```python
from build123d import *

# Parameters (mm, degrees)
F1_DEPTH      = 3
F2_DEPTH      = 6.85
F6_DEPTH      = 3
F3_W          = 16.2
F3_H          = 1
F7_DEPTH      = 1
F5_W          = 16.2
F5_H          = 1
F8_DEPTH      = 1
F4_W          = 1
F4_H          = 18.8
F9_DEPTH      = 1
F0_W          = 7
F0_H          = 10
F10_DEPTH     = 3
F11_D         = 8.2
F12_D         = 5
F13_R         = 0.6
F14_R         = 0.6
F15_T1_DEPTH  = 18
F15_S5_W      = 0.6
F15_S5_H      = 0.6
F15_T6_DEPTH  = 0.6
F15_S11_W     = 0.6
F15_S11_H     = 0.6
F15_T12_DEPTH = 0.6


# Not quite as in the source:
# - a fillet or chamfer that OpenCascade refuses, or shapes differently, is made with other operations: its cross-section is extruded or revolved along the edge and cut away or added
# - a feature names something its author has since deleted; it is built from what else it names


with BuildPart() as f1:
    # F0 (on Front) → F1 (new body)
    with BuildSketch(Plane.XZ):
        Polygon((0.9, 2.1), (4.9, 2.1), (21.1, 2.1), (21.1, 20.9), (4.9, 20.9), (0.9, 20.9), align=None)
        Polygon((4.9, 2.1), (4.9, 0), (7, 0), (15, 0), (22, 0), (22, 23), (15, 23), (7, 23), (4.9, 23), (4.9, 20.9), (21.1, 20.9), (21.1, 2.1), align=None)
    extrude(amount=F1_DEPTH)

    # F0 (on Front) → F2 (join)
    with BuildSketch(Plane.XZ):
        Polygon((4.9, 2.1), (4.9, 0), (7, 0), (15, 0), (22, 0), (22, 23), (15, 23), (7, 23), (4.9, 23), (4.9, 20.9), (21.1, 20.9), (21.1, 2.1), align=None)
    extrude(amount=F2_DEPTH)

    # F0 (on Front) → F6 (join)
    with BuildSketch(Plane.XZ):
        Polygon((0, 23), (0, 0), (4.9, 0), (4.9, 2.1), (0.9, 2.1), (0.9, 20.9), (4.9, 20.9), (4.9, 23), align=None)
    extrude(amount=F6_DEPTH)

    # F3 (on face) → F7 (join)
    with BuildSketch(Plane(origin=(0, 0, 20.9), x_dir=(1, 0, 0), z_dir=(0, 0, -1))):
        with Locations((13, 6.35)):
            Rectangle(F3_W, F3_H)
    extrude(amount=F7_DEPTH)

    # F5 (on face) → F8 (join)
    with BuildSketch(Plane.XY.offset(2.1)):
        with Locations((13, -6.35)):
            Rectangle(F5_W, F5_H)
    extrude(amount=F8_DEPTH)

    # F4 (on face) → F9 (join)
    with BuildSketch(Plane(origin=(21.1, 0, 0), x_dir=(0, -1, 0), z_dir=(-1, 0, 0))):
        with Locations((6.35, 11.5)):
            Rectangle(F4_W, F4_H)
    extrude(amount=F9_DEPTH)

    # F0 (on Front) → F10 (join)
    with BuildSketch(Plane.XZ):
        with Locations((18.5, 28)):
            Rectangle(F0_W, F0_H)
        with Locations((18.5, -5)):
            Rectangle(F0_W, F0_H)
        Polygon((0, 33), (0, 23), (4.9, 23), (7, 23), (7, 33), align=None)
        Polygon((4.9, 0), (0, 0), (0, -10), (7, -10), (7, 0), align=None)
    extrude(amount=F10_DEPTH)

    # F11 (through all)
    with Locations(Plane(origin=(0, 0, 0), x_dir=(1, 0, 0), z_dir=(0, 1, 0))):
        with Locations((11, -11.5)):
            Hole(F11_D / 2)

    # F12 (through all)
    with Locations(Plane(origin=(0, 0, 0), x_dir=(1, 0, 0), z_dir=(0, 1, 0))):
        with Locations((3.5, -28), (18.5, -28), (3.5, 5), (18.5, 5)):
            Hole(F12_D / 2)

    # F13
    f13_edges = [f1.edges().sort_by_distance(p)[0] for p in [
        (0, -3, 11.5),
        (3.5, -3, -10),
        (7, -3, -5),
        (3.5, -3, 33),
        (7, -3, 28),
    ]]
    fillet(f13_edges, radius=F13_R)

    # F14
    f14_edges = [f1.edges().sort_by_distance(p)[0] for p in [
        (22, -3, -5),
        (18.5, -3, -10),
        (15, -3, -5),
        (22, -4.925, 0),
        (22, -6.85, 11.5),
        (22, -4.925, 23),
        (22, -3, 28),
        (15, -3, 28),
        (18.5, -3, 33),
    ]]
    fillet(f14_edges, radius=F14_R)

    # F15: fillet of radius 0.6 on 2 edges, made by hand

    # F15_s2 → F15_t1 (cut)
    with BuildSketch(Plane.YZ.offset(3.4)):
        with BuildLine():
            ThreePointArc((-6.25, 23), (-6.6742640687, 22.8242640687), (-6.85, 22.4))
            Line((-6.85, 22.4), (-6.85, 23))
            Line((-6.85, 23), (-6.25, 23))
        make_face()
        with BuildLine():
            ThreePointArc((-6.85, 0.6), (-6.6742640687, 0.1757359313), (-6.25, 0))
            Line((-6.25, 0), (-6.85, 0))
            Line((-6.85, 0), (-6.85, 0.6))
        make_face()
    extrude(amount=F15_T1_DEPTH, mode=Mode.SUBTRACT)


with BuildPart() as f15_tool4:
    # F15_s5 → F15_t6 (new body)
    with BuildSketch(Plane.XZ.offset(6.25)):
        with Locations((21.7, 0.3)):
            Rectangle(F15_S5_W, F15_S5_H)
    extrude(amount=F15_T6_DEPTH)

    # F15_s7 → F15_t8 (revolve, cut)
    with BuildSketch(Plane(origin=(21.4, -6.25, 0.6), x_dir=(-0.7071067812, 0, 0.7071067812), z_dir=(0.7071067812, 0, 0.7071067812))):
        with BuildLine():
            ThreePointArc((0, -0.6), (0.6, 0), (0, 0.6))
            Line((0, 0.6), (0, -0.6))
        make_face()
    revolve(axis=Axis((21.4, -6.25, 0.6), (0, -1, 0)), mode=Mode.SUBTRACT)


with BuildPart() as f1_1:
    add(f1.part)

    # F15_t3: cut F15_tool4
    add(f15_tool4.part, mode=Mode.SUBTRACT)


with BuildPart() as f15_tool10:
    # F15_s11 → F15_t12 (new body)
    with BuildSketch(Plane.XY.offset(22.4)):
        with Locations((21.7, -6.55)):
            Rectangle(F15_S11_W, F15_S11_H)
    extrude(amount=F15_T12_DEPTH)

    # F15_s13 → F15_t14 (revolve, cut)
    with BuildSketch(Plane(origin=(21.4, -6.25, 22.4), x_dir=(-0.7071067812, 0.7071067812, 0), z_dir=(0.7071067812, 0.7071067812, 0))):
        with BuildLine():
            ThreePointArc((0, -0.6), (0.6, 0), (0, 0.6))
            Line((0, 0.6), (0, -0.6))
        make_face()
    revolve(axis=Axis((21.4, -6.25, 22.4), (0, 0, 1)), mode=Mode.SUBTRACT)


with BuildPart() as f1_2:
    add(f1_1.part)

    # F15_t9: cut F15_tool10
    add(f15_tool10.part, mode=Mode.SUBTRACT)


solid = f1_2.part
```
The model under review builds one solid part; all positions refer to its coordinate system, in mm. A direction names the side the tool comes from. Round coordinates to 2 decimals unless told otherwise and drop trailing zeros. Loops run counter-clockwise (first coordinate to the right, second up) from the corner with the lowest first, then second, coordinate; pieces in that order, holes last. Notation, with made-up numbers: (12, -21) - (60, -21) arc R19 ccw to (60, -10) - close; hole circle Ø5 at (75.25, 49.25). An arc over 180 degrees is marked (long way). Write each question's results on one line, items separated by ' | '. Start each with the question number.
Q1. Wall thickness on line 1 along X through (y, z) = (-0.7, 28); line 2 along Z through (x, y) = (18.5, -1.45); line 3 along Z through (x, y) = (12.25, -3.25): over which ranges is each line inside the solid? List them lowest first. Write a range as [from, to].
Q2. Tool access review of faces 1 (the flat face through (15, -1, -5)), 2 (the flat face through (13, -4, 20.9)), 3 (the flat face through (13, -4, 0)): name each direction out of +Z, -Z, +X, -X, +Y, -Y from which nothing blocks a thin tool from reaching the whole face with its end or side.
Q3. Draft analysis for pull direction X (two halves, no side actions). For faces 4 (the cylindrical face through (2, -2, 26)), 5 (the flat face through (12, -6, 19.9)), 6 (the flat face through (22, -2, 11)), state which applies: pulls with the +X half, pulls with the -X half, needs draft (parallel to the pull), parting line crosses it, or undercut.
Q4. Insertion check: P1, Ø0.5, axis at y = -6, z = 11, coming from the -X side; P2, Ø4.5, axis at x = 17, z = 27, coming from the -Y side; P3, Ø1.7, axis at x = 18, z = -5.5, coming from the -Y side; P4, Ø2.5, axis at y = -5, z = 21, coming from the -X side. Each pin has a flat end and moves straight along its axis. Give the tip position at first contact, or say it passes through.
Q5. Take a section at A-A on z = 11.5. Give the boundary of the cut face in (x, y), plus the area to 3 significant figures.
Q6. Take a section at C-C on z = 30. Give the boundary of the cut face in (x, y).
Q7. Take a section at D-D on x = 11. Give the boundary of the cut face in (y, z), plus the area to 3 significant figures.
Q8. Take a section at B-B on x = 18.5. Give the boundary of the cut face in (y, z).
Data:
1) line 1: x = [0, 1], [6, 7], [15, 16], [21, 22] | line 2: z = [-10, -7.5], [-2.5, 25.5], [30.5, 33] | line 3: z = [0, 2.1], [20.9, 23]
2) face 1: -Z, +Y, -Y | face 2: -X | face 3: -Z, -Y
3) face 4: undercut | face 5: needs draft | face 6: pulls with the +X half
4) P1: stops at x = 20.1 | P2: stops at y = -3 | P3: passes through | P4: stops at x = 4.9
5) outline: (0, -2.4) arc R0.6 ccw to (0.6, -3) - (6.9, -3) - (6.9, 0) - (0, 0) - close; (15.1, -3) - (21.1, -3) - (21.1, -5.85) - (20.1, -5.85) - (20.1, -6.85) - (21.4, -6.85) arc R0.6 ccw to (22, -6.25) - (22, 0) - (15.1, 0) - close | area: 45.7 mm²
6) outline: (0, -2.4) arc R0.6 ccw to (0.6, -3) - (2, -3) - (2, 0) - (0, 0) - close; (5, -3) - (6.4, -3) arc R0.6 ccw to (7, -2.4) - (7, 0) - (5, 0) - close; (15, -2.4) arc R0.6 ccw to (15.6, -3) - (17, -3) - (17, 0) - (15, 0) - close; (20, -3) - (21.4, -3) arc R0.6 ccw to (22, -2.4) - (22, 0) - (20, 0) - close
7) outline: (-6.85, 0.6) arc R0.6 ccw to (-6.25, 0) - (0, 0) - (0, 7.4) - (-3, 7.4) - (-3, 2.1) - (-5.85, 2.1) - (-5.85, 3.1) - (-6.85, 3.1) - close; (-6.85, 19.9) - (-5.85, 19.9) - (-5.85, 20.9) - (-3, 20.9) - (-3, 15.6) - (0, 15.6) - (0, 23) - (-6.25, 23) arc R0.6 ccw to (-6.85, 22.4) - close | area: 62.4 mm²
8) outline: (-6.85, 0.6) arc R0.6 ccw to (-6.25, 0) - (-3, 0) - (-3, -2.5) - (0, -2.5) - (0, 25.5) - (-3, 25.5) - (-3, 23) - (-6.25, 23) arc R0.6 ccw to (-6.85, 22.4) - (-6.85, 19.9) - (-5.85, 19.9) - (-5.85, 20.9) - (-3, 20.9) - (-3, 2.1) - (-5.85, 2.1) - (-5.85, 3.1) - (-6.85, 3.1) - close; (-3, -9.4) arc R0.6 ccw to (-2.4, -10) - (0, -10) - (0, -7.5) - (-3, -7.5) - close; (-3, 30.5) - (0, 30.5) - (0, 33) - (-2.4, 33) arc R0.6 ccw to (-3, 32.4) - close
